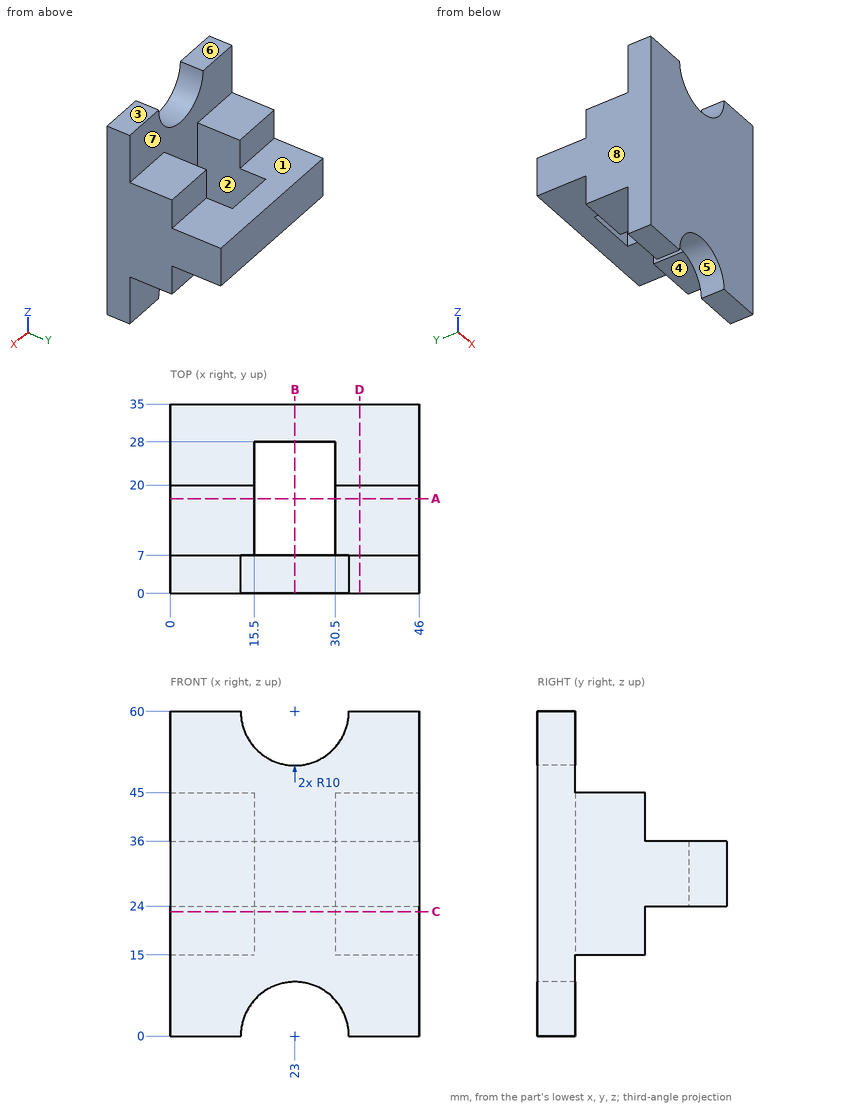
Source: three-view drawing plus pictorial views. Frame: mm from the lowest corner of the part. A direction names the side the tool comes from. Coordinates: 2 decimals unless noted, no trailing zeros. Loops run counter-clockwise (first coordinate to the right, second up) from the corner with the lowest first, then second, coordinate; pieces in that order, holes last. Notation, with made-up numbers: (52.5, 45.25) -> (82.5, 45.25) arc R17 ccw to (82.5, 76.25) -> close; hole circle Ø5 at (-17.5, -39.5). An arc over 180 degrees is marked (long way). Answer in a Markdown table with one row per item. Add a question column.
Q1. Ray query, line 1 along X through (y, z) = (24.5, 24.5); line 2 along Z through (x, y) = (12, 32); line 3 along Y through (x, z) = (25, 37). Return the intervals inside material, ascending.
Q2. Section A-A on y = 17.5. Return the cut outline in (x, z).
Q3. Reachability of the marked faces 1, 2, 3, 4 and 5 from +Z, -Z, +X, -X, +Y, -Y: full face, straight path, thin tool, end or side. Return the list, or none.
Q4. Section B-B on x = 23. Return the cut outline in (y, z), and give its area (3 significant figures).
Q5. Pull-direction query (X, two-part tool) for the marked faces 6, 7 and 8; classes: pulls with the +X half, pulls with the -X half, needs draft (parallel to the pull), parting line crosses it, or undercut.
Q6. Section D-D on x = 35. Return the cut outline in (y, z), and give its area (3 significant figures).
Q7. Section C-C on z = 23. Return the cut outline in (x, y).
Q8. Contact query for flat-ended pins moving along their axis: pin 1 Ø2.5 at (x, z) = (8.5, 19.5) entering from +Y; pin 2 Ø4 at (x, y) = (7, 14.5) entering from -Z; pin 3 Ø4 at (x, y) = (38.5, 16) entering from +Z. Output: stop coordinate, or through.
Computed values:
| question | item | result |
|---|---|---|
| 1 | line 1 | x = 0 to 15.5, 30.5 to 46 |
| 1 | line 2 | z = 24 to 36 |
| 1 | line 3 | y = 0 to 7 |
| 2 | outline | (0, 15) -> (15.5, 15) -> (15.5, 45) -> (0, 45) -> close; (30.5, 15) -> (46, 15) -> (46, 45) -> (30.5, 45) -> close |
| 3 | face 1 | +Z, +X, -X, +Y |
| 3 | face 2 | +Z, -Z |
| 3 | face 3 | +Z, +X, -X, +Y, -Y |
| 3 | face 4 | -Z, +X, -X, +Y |
| 3 | face 5 | -Z, +Y, -Y |
| 4 | outline | (0, 10) -> (7, 10) -> (7, 50) -> (0, 50) -> close; (28, 24) -> (35, 24) -> (35, 36) -> (28, 36) -> close |
| 4 | area | 364 mm^2 |
| 5 | face 6 | needs draft |
| 5 | face 7 | undercut |
| 5 | face 8 | pulls with the -X half |
| 6 | outline | (0, 0) -> (7, 0) -> (7, 15) -> (20, 15) -> (20, 24) -> (35, 24) -> (35, 36) -> (20, 36) -> (20, 45) -> (7, 45) -> (7, 60) -> (0, 60) -> close |
| 6 | area | 990 mm^2 |
| 7 | outline | (0, 0) -> (46, 0) -> (46, 20) -> (30.5, 20) -> (30.5, 7) -> (15.5, 7) -> (15.5, 20) -> (0, 20) -> close |
| 8 | pin 1 | stops at y = 20 |
| 8 | pin 2 | stops at z = 15 |
| 8 | pin 3 | stops at z = 45 |
